Design review of the part built by this model. Coordinates are the model's own, in mm. Face numbers are marked on the shaded views. A direction names the side the tool comes from. Coordinates: 2 decimals unless noted, no trailing zeros. Write each loop counter-clockwise with the first axis right and the second up, starting at its lowest first coordinate (ties: lowest second). Pieces come first, ordered by that corner, then holes. Notation, with made-up numbers: M 17,-15.75 L 70,-15.75 A25 ccw 70,5.25 Z; hole C 35,-12 d4. An arc over 180 degrees is marked long. Write item = value, one per line.
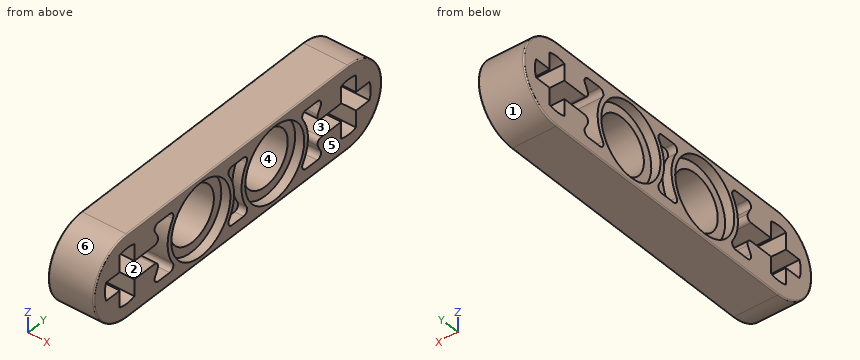
Autodesk Inventor part; units mm, degrees
ref_plane "YZ Plane" through (0, 0, 0) normal (1, 0, 0) x (0, 1, 0)
ref_plane "XZ Plane" through (0, 0, 0) normal (0, 1, 0) x (-1, 0, 0)
ref_plane "XY Plane" through (0, 0, 0) normal (0, 0, 1) x (1, 0, 0)
sketch "Sketch3" plane through (0, 0, 0) normal (1, 0, 0) x (0, 1, 0)
  arc A0 (12.8, 2.2627) -> (11.2, 2.2627) centre (12, 0) ccw
  arc A1 (11.2, -2.2627) -> (12.8, -2.2627) centre (12, 0) ccw
  arc A2 (14.2627, -0.8) -> (14.2627, 0.8) centre (12, 0) ccw
  line L0 (14.2627, 0.8) -> (12.8, 0.8)
  line L1 (11.2, 0.8) -> (8.49, 0.8)
  line L2 (12.8, 2.2627) -> (12.8, 0.8)
  line L3 (12.8, -0.8) -> (12.8, -2.2627)
  line L4 (14.2627, -0.8) -> (12.8, -0.8)
  line L5 (11.2, -0.8) -> (8.49, -0.8)
  arc A3 (12, -3.6) -> (12, 3.6) centre (12, 0) ccw
  line L6 (-12, -3.6) -> (12, -3.6)
  line L7 (-12, 3.6) -> (12, 3.6)
  line L8 (11.2, 0.8) -> (11.2, 2.2627)
  line L9 (11.2, -0.8) -> (11.2, -2.2627)
  arc A4 (-12, 3.6) -> (-12, -3.6) centre (-12, 0) ccw
  line L10 (0, -3.6) -> (0, 3.6) construction
  arc A5 (-11.2, 2.2627) -> (-12.8, 2.2627) centre (-12, 0) ccw
  arc A6 (-12.8, -2.2627) -> (-11.2, -2.2627) centre (-12, 0) ccw
  line L11 (-12.8, -0.8) -> (-12.8, -2.2627)
  line L12 (-12.8, 2.2627) -> (-12.8, 0.8)
  line L13 (-14.2627, -0.8) -> (-12.8, -0.8)
  line L14 (-14.2627, 0.8) -> (-12.8, 0.8)
  arc A7 (-14.2627, 0.8) -> (-14.2627, -0.8) centre (-12, 0) ccw
  line L15 (-11.2, 0.8) -> (-8.49, 0.8)
  line L16 (-11.2, -0.8) -> (-8.49, -0.8)
  line L17 (-11.2, 0.8) -> (-11.2, 2.2627)
  line L18 (-11.2, -0.8) -> (-11.2, -2.2627)
  circle A8 centre (-4, 0) radius 3.2
  circle A9 centre (4, 0) radius 3.2
  line L19 (12, 0) -> (4, 0) construction
  line L20 (4, 0) -> (-4, 0) construction
  line L21 (-4, 0) -> (-12, 0) construction
  circle A10 centre (-4, 0) radius 2.4
  circle A11 centre (4, 0) radius 2.4
  line L22 (-9.4544, 2.5456) -> (-6.5456, 2.5456)
  line L23 (-9.4544, -2.5456) -> (-6.5456, -2.5456)
  line L24 (-1.4544, 2.5456) -> (1.4544, 2.5456)
  line L25 (-1.4544, -2.5456) -> (1.4544, -2.5456)
  line L26 (6.5456, 2.5456) -> (9.4544, 2.5456)
  line L27 (6.5456, -2.5456) -> (9.4544, -2.5456)
  arc A12 (-9.4544, -2.5456) -> (-9.4544, 2.5456) centre (-12, 0) ccw
  arc A13 (-6.5456, 2.5456) -> (-6.5456, -2.5456) centre (-4, 0) ccw
  arc A14 (-1.4544, -2.5456) -> (-1.4544, 2.5456) centre (-4, 0) ccw
  arc A15 (1.4544, 2.5456) -> (1.4544, -2.5456) centre (4, 0) ccw
  arc A16 (6.5456, -2.5456) -> (6.5456, 2.5456) centre (4, 0) ccw
  arc A17 (9.4544, 2.5456) -> (9.4544, -2.5456) centre (12, 0) ccw
  line L28 (-12, 0) -> (-9.4544, 2.5456) construction
  arc A18 (8.49, 0.8) -> (8.49, -0.8) centre (12, 0) ccw
  point P0 (0, 0)
  dimension "d47" = 4.8
  dimension "d49" = 7.2
  dimension "d53" = 1.6
  dimension "d58" = 24
  dimension "d59" = 6.4
  dimension "d60" = 4.8
  dimension "d64" = 45
extrude "Extrusion4" add sketch "Sketch3" along normal mid plane 4 contours L6 A4 L7 A3 | A8 | A9 | L24 A15 L25 A14
sketch "Sketch11" plane through (2, 0, 0) normal (1, 0, 0) x (0, 0, -1)
  circle A0 centre (0, 4) radius 2.4
  circle A1 centre (0, -4) radius 2.4
  circle A2 centre (0, 4) radius 3.2
  circle A3 centre (0, -4) radius 3.2
  arc A4 (2.5456, 6.5456) -> (-2.5456, 6.5456) centre (0, 4) ccw
  arc A5 (-2.5456, -6.5456) -> (2.5456, -6.5456) centre (0, -4) ccw
  line L0 (-2.2627, -11.2) -> (-0.8, -11.2)
  line L1 (-2.5456, 1.4544) -> (-2.5456, -1.4544)
  line L2 (2.5456, 1.4544) -> (2.5456, -1.4544)
  arc A6 (-2.5456, 1.4544) -> (2.5456, 1.4544) centre (0, 4) ccw
  arc A7 (2.5456, -1.4544) -> (-2.5456, -1.4544) centre (0, -4) ccw
  point P0 (0, 0)
  dimension "d61" = 6.4
extrude "Extrusion16" cut sketch "Sketch11" against normal blind 0.8 contours A2 | A3
extrude "Extrusion17" cut sketch "Sketch11" against normal blind 0.8 contours A6 L2 A7 L1
mirror "Mirror3" about plane through (0, 0, 0) normal (1, 0, 0) of "Extrusion16", "Extrusion17"
fillet "Fillet1" radius 0.1 8 edges at (-2, 15.6, 0) (-2, 0, 3.6) (-2, 0, -3.6) (2, 0, 3.6) (2, 0, -3.6) (2, 15.6, 0) (-2, -15.6, 0) (2, -15.6, 0)
fillet "Fillet1" radius 0.4 20 edges at (0, -9.4544, 2.5456) (0, -6.5456, 2.5456) (0, -9.4544, -2.5456) (0, -6.5456, -2.5456) (1.6, -1.4544, -2.5456) (1.6, 1.4544, -2.5456) (1.6, 1.4544, 2.5456) (1.6, -1.4544, 2.5456) (0, 6.5456, 2.5456) (0, 9.4544, 2.5456) (0, 6.5456, -2.5456) (0, 9.4544, -2.5456) (-1.6, -1.4544, 2.5456) (-1.6, -1.4544, -2.5456) (-1.6, 1.4544, -2.5456) (-1.6, 1.4544, 2.5456) (0, -8.49, 0.8) (0, -8.49, -0.8) (0, 8.49, -0.8) (0, 8.49, 0.8)
equation "\"d47\" = kd"
equation "\"d49\" = tlad"
equation "\"d53\" = axlet"
equation "\"d58\" = 3 * lu"
equation "\"d59\" = tsd"
equation "\"d60\" = tpd"
equation "\"d15\" = 0.5 * lu"
equation "\"d61\" = tsd"
equation "\"d62\" = tsl"
equation "\"d65\" = 0.5 * lu - 2 * wall"
equation "\"lf\" = 0.1"
equation "\"tf\" = 0.4"
properties part number "32449-Yellow" material "ABS Plastic"
Q1. Wall thickness on line 1 (Y direction, x = 1.7, z = 0.25); line 2 (Y direction, x = -0.3, z = -2.5); line 3 (Y direction, x = 1.7, z = -0.5): over which ranges is each line inside the solid? List them lowest first.
Check result:
line_1 = -15.59 to -14.39, -7.59 to -7.19, -0.81 to -0.41, 0.41 to 0.81, 7.19 to 7.59, 14.39 to 15.59
line_2 = -14.59 to -8.81, -7.19 to 7.19, 8.81 to 14.59
line_3 = -15.57 to -14.35, -7.57 to -7.16, -0.84 to -0.43, 0.43 to 0.84, 7.16 to 7.57, 14.35 to 15.57
Q2. The part is to be moulded in two halves that separate along Y. For the marked faces 3, 4, 5 and 6, say which applies: +Y half, -Y half, draft (parallel to the pull), parting line (faces both ways), or undercut.
Check result:
face_3 = undercut
face_4 = undercut
face_5 = draft
face_6 = -Y half
Q3. For P1, Ø1.6, axis at x = -1, z = 1.5, coming from the -Y side, flat-tipped, find the tip position at first contact; note if it passes through.
Check result:
P1 = -15.53
Q4. Machinability: for the marked faces 1 and 2, which of the approach directions +Z, -Z, +X, -X, +Y, -Y give a long, thin tool a straight path to every point of the face, cutting with its end or side? Answer none if there is none.
Check result:
face_1 = +X, -X, +Y
face_2 = +X, -X
Q5. Consider section B-B, the plane z = 0. State how many separate pieces and enclosed holes the cut face has, and give its area (3 significant figures).
Check result:
separate_pieces = 5
enclosed_holes = 0
area = 25.6 mm²
Q6. Consider section A-A, the plane y = -4. State the section outline as (x, z) points, and give its area (3 significant figures).
Check result:
outline = M -2,-3.5 A0.1 ccw -1.9,-3.6 L 1.9,-3.6 A0.1 ccw 2,-3.5 L 2,-3.2 L 1.2,-3.2 L 1.2,-2.4 L -1.2,-2.4 L -1.2,-3.2 L -2,-3.2 Z; M -2,3.2 L -1.2,3.2 L -1.2,2.4 L 1.2,2.4 L 1.2,3.2 L 2,3.2 L 2,3.5 A0.1 ccw 1.9,3.6 L -1.9,3.6 A0.1 ccw -2,3.5 Z
area = 7.03 mm²
